Read the model definition and answer for the solid it produces. Units are mm, in the model's axes. A direction names the side the tool comes from. Coordinates: 2 decimals unless noted, no trailing zeros. Write each loop counter-clockwise with the first axis right and the second up, starting at its lowest first coordinate (ties: lowest second). Pieces come first, ordered by that corner, then holes. Notation, with made-up numbers: (5, 4) - (21, 4) arc R20 ccw to (21, 38) - close; hole circle Ø3 at (77, -5). An arc over 180 degrees is marked (long way). Use a Markdown table: item, result.
from build123d import *

# Parameters (mm, degrees)
SKETCH_1_W          = 36.5
SKETCH_1_H          = 18.8
EXTRUDE_1_DEPTH     = 22.5
FILLET_1_R          = 3
SKETCH_2_R          = 2.6
CUT_EXTRUDE_1_DEPTH = 35.536249073
SKETCH_3_W          = 2.4
SKETCH_3_H          = 5
EXTRUDE_2_DEPTH     = 5
SKETCH_4_R          = 1.4
CUT_EXTRUDE_2_DEPTH = 35.046622446
EXTRUDE_3_DEPTH     = 12
EXTRUDE_4_DEPTH     = 13
FILLET_2_R          = 3
EXTRUDE_5_DEPTH     = 3
SKETCH_9_R          = 2
EXTRUDE_7_DEPTH     = 21.05
SKETCH_10_W         = 2
SKETCH_10_H         = 5
EXTRUDE_8_DEPTH     = 12.5
SKETCH_11_R         = 1.5
CUT_EXTRUDE_3_DEPTH = 56.901006252


with BuildPart() as part:
    # 草图1 → 凸台-拉伸1 (new body)
    with BuildSketch(Plane(origin=(0, 0, 0), x_dir=(1, 0, 0), z_dir=(0, 1, 0))):
        Rectangle(SKETCH_1_W, SKETCH_1_H)
    extrude(amount=EXTRUDE_1_DEPTH)

    # 圆角1
    fillet_1_edges = [part.edges().sort_by_distance(p)[0] for p in [
        (-18.25, 22.5, 0),
        (-18.25, 0, 0),
    ]]
    fillet(fillet_1_edges, radius=FILLET_1_R)

    # 草图2 → 切除-拉伸1 (cut, through all)
    with BuildSketch(Plane.XY.offset(9.4)):
        with Locations((-8.25, 11.25)):
            Circle(SKETCH_2_R)
    extrude(amount=-CUT_EXTRUDE_1_DEPTH, mode=Mode.SUBTRACT)

    # 草图3 → 凸台-拉伸2 (add)
    with BuildSketch(Plane.ZY.offset(18.25)):
        with Locations((0, 11.25)):
            Rectangle(SKETCH_3_W, SKETCH_3_H)
    extrude(amount=EXTRUDE_2_DEPTH)

    # 草图4 → 切除-拉伸2 (cut, through all)
    with BuildSketch(Plane.XY.offset(1.2)):
        with Locations((-20.559983935, 11.316362833)):
            Circle(SKETCH_4_R)
    extrude(amount=-CUT_EXTRUDE_2_DEPTH, mode=Mode.SUBTRACT)

    # 草图5 → 凸台-拉伸3 (add)
    with BuildSketch(Plane(origin=(18.25, 0, 0), x_dir=(0, 0, -1), z_dir=(1, 0, 0))):
        with BuildLine():
            Line((-9.4, 18.083062757), (-9.4, 4.416937243))
            ThreePointArc((-9.4, 4.416937243), (-9.262387752, 3.78932302), (-8.874800516, 3.276865335))
            ThreePointArc((-8.874800516, 3.276865335), (0, 0), (8.874800516, 3.276865335))
            ThreePointArc((8.874800516, 3.276865335), (9.262387752, 3.78932302), (9.4, 4.416937243))
            Line((9.4, 4.416937243), (9.4, 18.083062757))
            ThreePointArc((9.4, 18.083062757), (9.262387752, 18.71067698), (8.874800516, 19.223134665))
            ThreePointArc((8.874800516, 19.223134665), (0, 22.5), (-8.874800516, 19.223134665))
            ThreePointArc((-8.874800516, 19.223134665), (-9.262387752, 18.71067698), (-9.4, 18.083062757))
        make_face()
    extrude(amount=EXTRUDE_3_DEPTH)

    # 草图6 → 凸台-拉伸4 (add)
    with BuildSketch(Plane(origin=(30.25, 0, 0), x_dir=(0, 0, -1), z_dir=(1, 0, 0))):
        with BuildLine():
            Line((-8.4, 17.356141187), (-8.4, 5.143858813))
            ThreePointArc((-8.4, 5.143858813), (0, 1.003858813), (8.4, 5.143858813))
            Line((8.4, 5.143858813), (8.4, 17.356141187))
            ThreePointArc((8.4, 17.356141187), (0, 21.496141187), (-8.4, 17.356141187))
        make_face()
    extrude(amount=EXTRUDE_4_DEPTH)

    # 圆角2
    fillet_2_edges = [part.edges().sort_by_distance(p)[0] for p in [
        (36.75, 5.143858813, 8.4),
        (36.75, 5.143858813, -8.4),
        (36.75, 17.356141187, -8.4),
        (36.75, 17.356141187, 8.4),
    ]]
    fillet(fillet_2_edges, radius=FILLET_2_R)

    # 圆角3: read off the stored shape, not the designer's step
    # 圆角3 outline → 圆角3 (revolve, cut)
    with BuildSketch(Plane(origin=(0, 10.904402057, 0), x_dir=(0, 1, 0), z_dir=(0, 0, -1))):
        with BuildLine():
            ThreePointArc((6.59173913, 43.25), (9.420166255, 42.078427125), (10.59173913, 39.25))
            Line((10.59173913, 39.25), (10.59173913, 43.25))
            Line((10.59173913, 43.25), (6.59173913, 43.25))
        make_face()
    revolve(axis=Axis((0, 10.904402057, 0), (1, 0, 0)), mode=Mode.SUBTRACT)

    # 草图7 → 凸台-拉伸5 (add)
    with BuildSketch(Plane(origin=(43.25, 0, 0), x_dir=(0, 0, -1), z_dir=(1, 0, 0))):
        with BuildLine():
            Line((2.645751311, 7.904402057), (2.645751311, 13.904402057))
            ThreePointArc((2.645751311, 13.904402057), (-4, 10.904402057), (2.645751311, 7.904402057))
        make_face()
    extrude(amount=EXTRUDE_5_DEPTH)

    # 草图9 → 凸台-拉伸7 (add)
    with BuildSketch(Plane(origin=(0, 0, -9.4), x_dir=(-1, 0, 0), z_dir=(0, 0, -1))):
        with Locations((-3.25, 11.25)):
            Circle(SKETCH_9_R)
    extrude(amount=-EXTRUDE_7_DEPTH)

    # 草图10 → 凸台-拉伸8 (add, symmetric)
    with BuildSketch(Plane.XY):
        with Locations((24.25, 11.25)):
            Rectangle(SKETCH_10_W, SKETCH_10_H)
    extrude(amount=EXTRUDE_8_DEPTH, both=True)

    # 草图11 → 切除-拉伸3 (cut, through all)
    with BuildSketch(Plane.XY.offset(9.4)):
        with Locations((13.75, 15.5)):
            Circle(SKETCH_11_R)
    extrude(amount=-CUT_EXTRUDE_3_DEPTH, mode=Mode.SUBTRACT)


solid = part.part
(1) Each of these flat-tipped pins is pushed along its axis until it touches: P1, Ø5.5, axis at x = -20, y = 10.5, coming from the +Z side; P2, Ø2, axis at x = 24, z = 11, coming from the +Y side; P3, Ø6, axis at x = 13, y = 13.5, coming from the -Z side. Where does it stop, or does it pass through?
Report:
| item | result |
|---|---|
| P1 | stops at z = 9.4 |
| P2 | stops at y = 13.75 |
| P3 | stops at z = -9.4 |
(2) For faces 1 (the flat face through (18.25, 1, -7)), 2 (the flat face through (25.25, 11, -11)), 3 (the cylindrical face through (36.15, 5.13, 8.18)), 4 (the flat face through (24, 13.75, 11)), determine the directions among +Z, -Z, +X, -X, +Y, -Y from which every point of the face is accessible in a straight line to the end or side of a thin tool.
Report:
| item | result |
|---|---|
| face 1 | -Z, +X, -Y |
| face 2 | -Z, +X, +Y, -Y |
| face 3 | +Z, +X, -Y |
| face 4 | +Z, +X, -X, +Y |
(3) The mould has two halves that part along Y. Classify faces 5 (the cylindrical face through (-21.592, 12.263, 0.017)), 6 (the cylindrical face through (35.91, 17.37, 8.18)), 7 (the flat face through (-23.25, 11, 0)), 8 (the cylindrical face through (-8.81, 8.71, 0.13)): pulls with the +Y half, pulls with the -Y half, needs draft (parallel to the pull), parting line crosses it, or undercut.
Report:
| item | result |
|---|---|
| face 5 | undercut |
| face 6 | pulls with the +Y half |
| face 7 | needs draft |
| face 8 | undercut |
(4) A cutting plane is placed at B-B, the plane x = 3.25. Write down the section's boundary in (y, z), and give its area (3 significant figures).
Report:
| item | result |
|---|---|
| outline | (0, -9.4) - (22.5, -9.4) - (22.5, 9.4) - (13.25, 9.4) - (13.25, 11.65) - (9.25, 11.65) - (9.25, 9.4) - (0, 9.4) - close |
| area | 432 mm² |
(5) Straight lines are drawn through the part: L1, parallel to Y at x = 13.75, z = -5.5; L2, parallel to Y at x = -8.25, z = 4.5; L3, parallel to Y at x = -15.5, z = -2.75. For each, find the intervals that lie inside material, in ascending order.
Report:
| item | result |
|---|---|
| L1 | y = 0 to 14, 17 to 22.5 |
| L2 | y = 0 to 8.65, 13.85 to 22.5 |
| L3 | y = 0.01 to 22.49 |
(6) A cutting plane is placed at A-A, the plane x = -8.25. Write down the section's boundary in (y, z).
Report:
| item | result |
|---|---|
| outline | (0, -9.4) - (8.65, -9.4) - (8.65, 9.4) - (0, 9.4) - close; (13.85, -9.4) - (22.5, -9.4) - (22.5, 9.4) - (13.85, 9.4) - close |
(7) A cutting plane is placed at D-D, the plane z = 3.25. Count the separate pieces of the cut face and the enclosed holes in it, and give its area (3 significant figures).
Report:
| item | result |
|---|---|
| separate pieces | 1 |
| enclosed holes | 2 |
| area | 1,310 mm² |
(8) A cutting plane is placed at C-C, the plane x = 13.75. Write down the section's boundary in (y, z), and give its area (3 significant figures).
Report:
| item | result |
|---|---|
| outline | (0, -9.4) - (14, -9.4) - (14, 9.4) - (0, 9.4) - close; (17, -9.4) - (22.5, -9.4) - (22.5, 9.4) - (17, 9.4) - close |
| area | 367 mm² |
